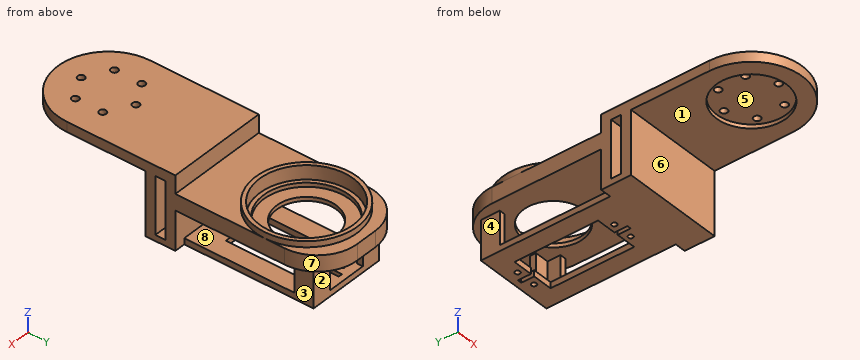
from build123d import *

# Parameters (mm, degrees)
EXTRUDE_1_DEPTH     = 5
SKETCH_2_R          = 17.5
CUT_EXTRUDE_1_DEPTH = 2
SKETCH_3_R          = 1.75
CUT_EXTRUDE_2_DEPTH = 61.245331769
SKETCH_4_W          = 51
SKETCH_4_H          = 5
EXTRUDE_2_DEPTH     = 31.7
SKETCH_12_W         = 51
SKETCH_12_H         = 8
EXTRUDE_7_DEPTH     = 75
FILLET_2_R          = 20
CUT_EXTRUDE_6_REACH = 135.449
SKETCH_13_R         = 15
SKETCH_14_R         = 25.5
EXTRUDE_8_DEPTH     = 3
SKETCH_16_R         = 23.5
CUT_EXTRUDE_7_DEPTH = 7
SKETCH_17_R         = 21.5
CUT_EXTRUDE_8_DEPTH = 2
EXTRUDE_9_DEPTH     = 19.7
EXTRUDE_10_DEPTH    = 3
CUT_EXTRUDE_9_REACH = 138.994
SKETCH_20_R         = 1.25


with BuildPart() as part:
    # 스케치1 → 보스-돌출1 (new body)
    with BuildSketch(Plane.XY):
        with BuildLine():
            Line((-25.5, 0), (-25.5, 54.5))
            Line((-25.5, 54.5), (25.5, 54.5))
            Line((25.5, 54.5), (25.5, 0))
            ThreePointArc((25.5, 0), (0, -25.5), (-25.5, 0))
        make_face()
    extrude(amount=EXTRUDE_1_DEPTH)

    # 스케치2 → 컷-돌출1 (cut)
    with BuildSketch(Plane(origin=(0, 0, 0), x_dir=(-1, 0, 0), z_dir=(0, 0, -1))):
        Circle(SKETCH_2_R)
    extrude(amount=-CUT_EXTRUDE_1_DEPTH, mode=Mode.SUBTRACT)

    # 스케치3 → 컷-돌출2 (cut, through all)
    with BuildSketch(Plane(origin=(0, 0, 2), x_dir=(-1, 0, 0), z_dir=(0, 0, -1))):
        with Locations((0, 13.75)):
            Circle(SKETCH_3_R)
        with Locations((11.907849302, 6.875)):
            Circle(SKETCH_3_R)
        with Locations((11.907849302, -6.875)):
            Circle(SKETCH_3_R)
        with Locations((0, -13.75)):
            Circle(SKETCH_3_R)
        with Locations((-11.907849302, -6.875)):
            Circle(SKETCH_3_R)
        with Locations((-11.907849302, 6.875)):
            Circle(SKETCH_3_R)
    extrude(amount=-CUT_EXTRUDE_2_DEPTH, mode=Mode.SUBTRACT)

    # 스케치4 → 보스-돌출2 (add)
    with BuildSketch(Plane(origin=(0, 0, 0), x_dir=(-1, 0, 0), z_dir=(0, 0, -1))):
        with Locations((0, 52)):
            Rectangle(SKETCH_4_W, SKETCH_4_H)
        with Locations((0, 42)):
            Rectangle(SKETCH_4_W, SKETCH_4_H)
    extrude(amount=EXTRUDE_2_DEPTH)

    # 스케치12 → 보스-돌출7 (add)
    with BuildSketch(Plane(origin=(0, 54.5, 0), x_dir=(1, 0, 0), z_dir=(0, 1, 0))):
        with Locations((0, 8)):
            Rectangle(SKETCH_12_W, SKETCH_12_H)
    extrude(amount=EXTRUDE_7_DEPTH)

    # 필렛2
    fillet_2_edges = [part.edges().sort_by_distance(p)[0] for p in [
        (-25.5, 129.5, -8),
        (25.5, 129.5, -8),
    ]]
    fillet(fillet_2_edges, radius=FILLET_2_R)

    # 스케치13 → 컷-돌출6 (cut, up to next)
    with BuildSketch(Plane(origin=(0, 0, -12), x_dir=(-1, 0, 0), z_dir=(0, 0, -1)), mode=Mode.PRIVATE) as cut_extrude_6_sk1:
        with Locations((0, 99.5)):
            Circle(SKETCH_13_R)
    cut_extrude_6_tool1 = extrude(cut_extrude_6_sk1.sketch, amount=-CUT_EXTRUDE_6_REACH, mode=Mode.PRIVATE) & part.part
    add(cut_extrude_6_tool1.solids().sort_by_distance((0, 99.5, -12))[0], mode=Mode.SUBTRACT)

    # 스케치14 → 보스-돌출8 (add)
    with BuildSketch(Plane.XY.offset(-4)):
        with Locations((0, 99.5)):
            Circle(SKETCH_14_R)
    extrude(amount=EXTRUDE_8_DEPTH)

    # 스케치16 → 컷-돌출7 (cut)
    with BuildSketch(Plane.XY.offset(-1)):
        with Locations((0, 99.5)):
            Circle(SKETCH_16_R)
    extrude(amount=-CUT_EXTRUDE_7_DEPTH, mode=Mode.SUBTRACT)

    # 스케치17 → 컷-돌출8 (cut)
    with BuildSketch(Plane.XY.offset(-8)):
        with Locations((0, 99.5)):
            Circle(SKETCH_17_R)
    extrude(amount=-CUT_EXTRUDE_8_DEPTH, mode=Mode.SUBTRACT)

    # 스케치18 → 보스-돌출9 (add)
    with BuildSketch(Plane(origin=(0, 0, -12), x_dir=(-1, 0, 0), z_dir=(0, 0, -1))):
        Polygon((-20, 119.5), (-10, 119.5), (-10, 116.5), (-17, 116.5), (-17, 110), (-20, 110), align=None)
        Polygon((20, 119.5), (10, 119.5), (10, 116.5), (17, 116.5), (17, 110), (20, 110), align=None)
    extrude(amount=EXTRUDE_9_DEPTH)

    # 스케치19 → 보스-돌출10 (add)
    with BuildSketch(Plane(origin=(0, 0, -31.7), x_dir=(-1, 0, 0), z_dir=(0, 0, -1))):
        Polygon((-20, 119.5), (20, 119.5), (20, 54.5), (25.5, 54.5), (25.5, 39.5), (-25.5, 39.5), (-25.5, 54.5), (-20, 54.5), align=None)
    extrude(amount=-EXTRUDE_10_DEPTH)

    # 스케치20 → 컷-돌출9 (cut, up to next)
    with BuildSketch(Plane(origin=(0, 0, -31.7), x_dir=(-1, 0, 0), z_dir=(0, 0, -1)), mode=Mode.PRIVATE) as cut_extrude_9_sk1:
        with Locations((-5, 113.35)):
            Circle(SKETCH_20_R)
    cut_extrude_9_tool1 = extrude(cut_extrude_9_sk1.sketch, amount=-CUT_EXTRUDE_9_REACH, mode=Mode.PRIVATE) & part.part
    # 스케치20 → 컷-돌출9 (cut, up to next)
    with BuildSketch(Plane(origin=(0, 0, -31.7), x_dir=(-1, 0, 0), z_dir=(0, 0, -1)), mode=Mode.PRIVATE) as cut_extrude_9_sk2:
        with Locations((5, 113.35)):
            Circle(SKETCH_20_R)
    cut_extrude_9_tool2 = extrude(cut_extrude_9_sk2.sketch, amount=-CUT_EXTRUDE_9_REACH, mode=Mode.PRIVATE) & part.part
    # 스케치20 → 컷-돌출9 (cut, up to next)
    with BuildSketch(Plane(origin=(0, 0, -31.7), x_dir=(-1, 0, 0), z_dir=(0, 0, -1)), mode=Mode.PRIVATE) as cut_extrude_9_sk3:
        with Locations((-5, 64.75)):
            Circle(SKETCH_20_R)
    cut_extrude_9_tool3 = extrude(cut_extrude_9_sk3.sketch, amount=-CUT_EXTRUDE_9_REACH, mode=Mode.PRIVATE) & part.part
    # 스케치20 → 컷-돌출9 (cut, up to next)
    with BuildSketch(Plane(origin=(0, 0, -31.7), x_dir=(-1, 0, 0), z_dir=(0, 0, -1)), mode=Mode.PRIVATE) as cut_extrude_9_sk4:
        with Locations((5, 64.75)):
            Circle(SKETCH_20_R)
    cut_extrude_9_tool4 = extrude(cut_extrude_9_sk4.sketch, amount=-CUT_EXTRUDE_9_REACH, mode=Mode.PRIVATE) & part.part
    # 스케치20 → 컷-돌출9 (cut, up to next)
    with BuildSketch(Plane(origin=(0, 0, -31.7), x_dir=(-1, 0, 0), z_dir=(0, 0, -1)), mode=Mode.PRIVATE) as cut_extrude_9_sk5:
        Polygon((1, 110), (11, 110), (11, 68), (1, 68), (1, 61.5), (-1, 61.5), (-1, 68), (-11, 68), (-11, 110), (-1, 110), (-1, 116.5), (1, 116.5), align=None)
    cut_extrude_9_tool5 = extrude(cut_extrude_9_sk5.sketch, amount=-CUT_EXTRUDE_9_REACH, mode=Mode.PRIVATE) & part.part
    add(cut_extrude_9_tool1.solids().sort_by_distance((5, 113.35, -31.7))[0], mode=Mode.SUBTRACT)
    add(cut_extrude_9_tool2.solids().sort_by_distance((-5, 113.35, -31.7))[0], mode=Mode.SUBTRACT)
    add(cut_extrude_9_tool3.solids().sort_by_distance((5, 64.75, -31.7))[0], mode=Mode.SUBTRACT)
    add(cut_extrude_9_tool4.solids().sort_by_distance((-5, 64.75, -31.7))[0], mode=Mode.SUBTRACT)
    add(cut_extrude_9_tool5.solids().sort_by_distance((0, 89, -31.7))[0], mode=Mode.SUBTRACT)


solid = part.part
The model under review builds one solid part; all positions refer to its coordinate system, in mm. Face numbers are marked on the shaded views. A direction names the side the tool comes from. Round coordinates to 2 decimals unless told otherwise and drop trailing zeros. Order: outer loops, then holes, each group sorted by start corner. A loop starts at its lowest first (then second) coordinate and runs counter-clockwise, first axis right, second up. Notation, with made-up numbers: (9, 65) -> (18, 65) arc R21 cw to (18, 104) -> close; hole circle Ø4 at (18, 43.5). An arc over 180 degrees is marked (long way). Return JSON: item names as keys, results as strings.
1. Take a section at A-A (z = -6.5). Write out the cut boundary in (x, y).
Answer block:
{"outline": "(-25.5, 39.5) -> (25.5, 39.5) -> (25.5, 44.5) -> (-25.5, 44.5) -> close; (-25.5, 49.5) -> (25.5, 49.5) -> (25.5, 109.5) arc R20 ccw to (5.5, 129.5) -> (-5.5, 129.5) arc R20 ccw to (-25.5, 109.5) -> close; hole circle Ø47 at (0, 99.5)"}
2. For L1, parallel to Y at x = 5, z = -29; L2, parallel to Y at x = 0, z = 3; L3, parallel to Y at x = -16, z = -17, list the stretches that pass through material, from the lowest coordinate up. Write a range as [from, to].
Answer block:
{"L1": "y = [39.5, 63.5], [66, 68], [110, 112.1], [114.6, 119.5]", "L2": "y = [-25.5, -15.5], [-12, 12], [15.5, 54.5]", "L3": "y = [39.5, 44.5], [49.5, 54.5], [116.5, 119.5]"}
3. For the marked faces 1, 2, 3, 4 and 5, list the 3-axis set-ups (+Z, -Z, +X, -X, +Y, -Y) from which the entire face can be reached by the end or side of a thin tool; tool diameter is ignored.
Answer block:
{"face 1": "-Z, +X, -X, -Y", "face 2": "-Z, +X, -X, +Y", "face 3": "-Z, +X, +Y", "face 4": "-Z, -X, +Y", "face 5": "-Z"}
4. Insertion check: P1, Ø1.5, axis at y = 64.5, z = -30.5, coming from the +X side; P2, Ø4, axis at x = 9, z = -12, coming from the -Y side; P3, Ø4, axis at x = 5, y = 64.75, coming from the -Z side; P4, Ø2.5, axis at y = 118.5, z = -24, coming from the -X side. Each pin has a flat end and moves straight along its axis. Give the tip position at first contact, or say it passes through.
Answer block:
{"P1": "stops at x = 20", "P2": "stops at y = 39.5", "P3": "stops at z = -31.7", "P4": "stops at x = -20"}
5. Take a section at D-D (y = 86). Write out the cut boundary in (x, z).
Answer block:
{"outline": "(-25.5, -12) -> (-6.54, -12) -> (-6.54, -10) -> (-16.73, -10) -> (-16.73, -8) -> (-19.24, -8) -> (-19.24, -1) -> (-21.63, -1) -> (-21.63, -4) -> (-25.5, -4) -> close; (-20, -31.7) -> (-11, -31.7) -> (-11, -28.7) -> (-20, -28.7) -> close; (6.54, -12) -> (25.5, -12) -> (25.5, -4) -> (21.63, -4) -> (21.63, -1) -> (19.24, -1) -> (19.24, -8) -> (16.73, -8) -> (16.73, -10) -> (6.54, -10) -> close; (11, -31.7) -> (20, -31.7) -> (20, -28.7) -> (11, -28.7) -> close"}
6. Take a section at B-B (y = -13.75). Write out the cut boundary in (x, z).
Answer block:
{"outline": "(-21.48, 0) -> (-10.83, 0) -> (-10.83, 2) -> (-1.75, 2) -> (-1.75, 5) -> (-21.48, 5) -> close; (1.75, 2) -> (10.83, 2) -> (10.83, 0) -> (21.48, 0) -> (21.48, 5) -> (1.75, 5) -> close"}
7. The part is to be moulded in two halves that separate along X. For the marked faces 6, 7 and 8, say which applies: +X half, -X half, draft (parallel to the pull), parting line (faces both ways), or undercut.
Answer block:
{"face 6": "draft", "face 7": "+X half", "face 8": "undercut"}
8. Take a section at C-C (x = 8). State how many separate pieces and enclosed holes the cut face has, then the cut area to 3 significant figures.
Answer block:
{"separate pieces": "3", "enclosed holes": "1", "area": "1,040 mm²"}
